Solid Edge part; units mm, degrees
sketch "Sketch1" plane through (0, 0, 0) normal (0, 0, 1) x (1, 0, 0)
  line L0 (-6.1009, 4.0673) -> (-6.5728, -3.2499)
  line L1 (-6.5728, -3.2499) -> (-0.4719, -7.3171)
  line L2 (-0.4719, -7.3171) -> (6.1009, -4.0673)
  line L3 (6.1009, -4.0673) -> (6.5728, 3.2499)
  line L4 (6.5728, 3.2499) -> (0.4719, 7.3171)
  line L5 (0.4719, 7.3171) -> (-6.1009, 4.0673)
extrude "Protrusion1" add sketch "Sketch1" against normal blind 105
sketch "Sketch2" plane through (0, 0, -2) normal (0, 0, 1) x (-0.8964, -0.4432, 0)
  circle A0 centre (0, 0) radius 5.5
  circle A1 centre (0, 0) radius 13.1424
extrude "ExtrudedCutout_1" cut sketch "Sketch2" against normal blind 2
sketch "Sketch3" plane through (0, 0, -103) normal (0, 0, -1) x (0.8964, 0.4432, 0)
  circle A0 centre (0, 0) radius 5.5
  circle A1 centre (0, 0) radius 13.1424
extrude "ExtrudedCutout_2" cut sketch "Sketch3" against normal blind 2
properties part number "BumbleB0505"
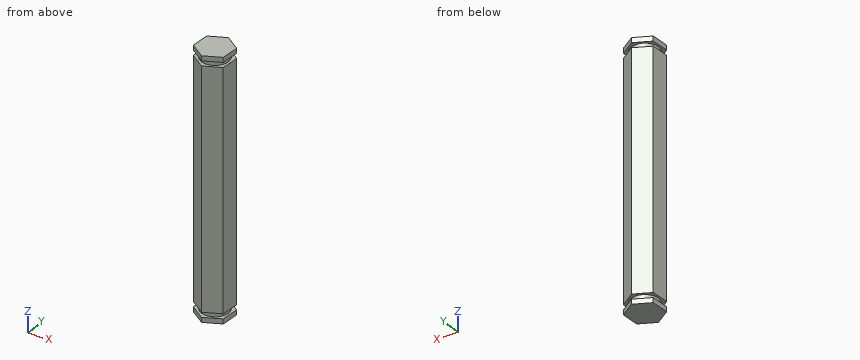
Build history of the part. All positions in model axes, mm. Round coordinates to 2 decimals unless told otherwise and drop trailing zeros. Write each loop counter-clockwise with the first axis right and the second up, starting at its lowest first coordinate (ties: lowest second). Pieces come first, ordered by that corner, then holes.
1) Drill centre lines: probe 1 along Z at (x, y) = (3.5, -5); probe 2 along Y at (x, z) = (4.5, -74.5); probe 3 along Y at (x, z) = (-4.25, -67). Where is each one in solid material? Low to high.
2) Band-saw the part on A-A, the plane x = 2.25. List the corners of the cut face in (y, z), and give its area (3 significant figures).
3) Pin check, flat tips, straight feed: pin 1 (4 mm diameter, centred on x = 0.5, y = 0, fed in from +Z); pin 2 (1 mm diameter, centred on y = 1.5, z = -80, fed in from +X). Stop position of each tip, or through.
4) Band-saw the part on C-C, the plane y = 0. List the corners of the cut face in (x, z), and give its area (3 significant figures).
5) Band-saw the part on B-B, the plane z = -56.5. List the corners of the cut face in (x, y).
Ans:
1. probe 1: z = -105 to -103, -101 to -4, -2 to 0
1. probe 2: y = -4.86 to 4.63
1. probe 3: y = -4.8 to 4.98
2. outline: (-5.97, -105) - (6.13, -105) - (6.13, -103) - (5.02, -103) - (5.02, -101) - (6.13, -101) - (6.13, -4) - (5.02, -4) - (5.02, -2) - (6.13, -2) - (6.13, 0) - (-5.97, 0) - (-5.97, -2) - (-5.02, -2) - (-5.02, -4) - (-5.97, -4) - (-5.97, -101) - (-5.02, -101) - (-5.02, -103) - (-5.97, -103) - close
2. area: 1,260 mm2
3. pin 1: stops at z = 0
3. pin 2: stops at x = 6.49
4. outline: (-6.36, -105) - (6.36, -105) - (6.36, -103) - (5.5, -103) - (5.5, -101) - (6.36, -101) - (6.36, -4) - (5.5, -4) - (5.5, -2) - (6.36, -2) - (6.36, 0) - (-6.36, 0) - (-6.36, -2) - (-5.5, -2) - (-5.5, -4) - (-6.36, -4) - (-6.36, -101) - (-5.5, -101) - (-5.5, -103) - (-6.36, -103) - close
4. area: 1,330 mm2
5. outline: (-6.57, -3.25) - (-0.47, -7.32) - (6.1, -4.07) - (6.57, 3.25) - (0.47, 7.32) - (-6.1, 4.07) - close
